Input: dimensioned drawing with shaded views. Units: mm. Origin: part minimum x, y, z. Coordinates: 2 decimals unless noted, no trailing zeros. Write each loop counter-clockwise with the first axis right and the second up, starting at its lowest first coordinate (ties: lowest second). Pieces come first, ordered by that corner, then holes. Notation, with made-up numbers: (-27.5, 54) - (19.5, 54) arc R32 ccw to (19.5, 86) - close; hole circle Ø6 at (-31.75, 84). An arc over 180 degrees is marked (long way). One line per question, with ' | ' between items.
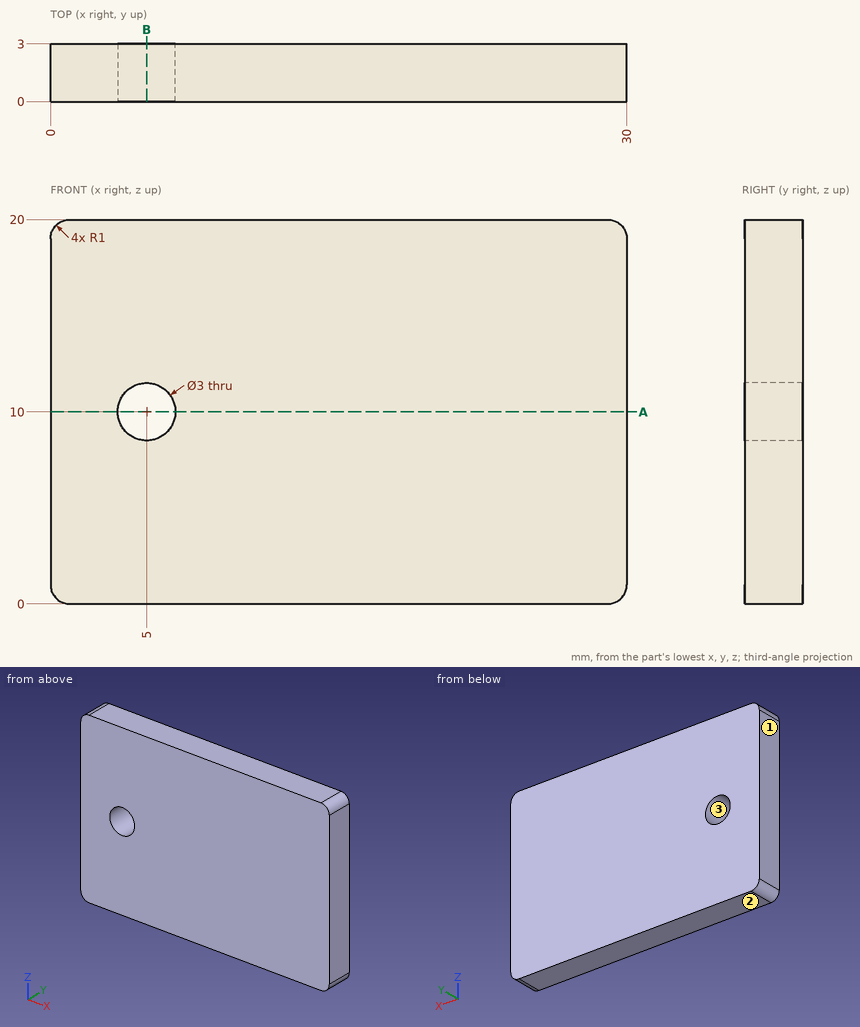
Item 1: Cut plane A-A on z = 10. Return loops of the section in (x, y).
Check sheet entries:
outline: (0, 0) - (3.5, 0) - (3.5, 3) - (0, 3) - close; (6.5, 0) - (30, 0) - (30, 3) - (6.5, 3) - close
Item 2: Mould query, pull axis X, two halves, no side actions, for the marked faces 1, 2 and 3. Classes: pulls with the +X half, pulls with the -X half, needs draft (parallel to the pull), parting line crosses it, or undercut.
Check sheet entries:
face 1: pulls with the -X half | face 2: needs draft | face 3: undercut
Item 3: Pin query (flat end, axial travel): pin 1 Ø5 at (x, z) = (5, 10) entering from -Y. Return the tip coordinate at first contact, or that it passes through.
Check sheet entries:
pin 1: y = 0
Item 4: Cut plane B-B on x = 5. Return loops of the section in (y, z), and give its area (3 significant figures).
Check sheet entries:
outline: (0, 0) - (3, 0) - (3, 8.5) - (0, 8.5) - close; (0, 11.5) - (3, 11.5) - (3, 20) - (0, 20) - close | area: 51.0 mm²
Item 5: Ray query, line 1 along Z through (x, y) = (5, 1.2); line 2 along X through (y, z) = (1.45, 10); line 3 along Z through (x, y) = (4.25, 0.8). Return the intervals inside material, ascending. Write a range as [from, to].
Check sheet entries:
line 1: [0, 8.5], [11.5, 20] | line 2: [0, 3.5], [6.5, 30] | line 3: [0, 8.7], [11.3, 20]
